Build history of the part. All positions in model axes, mm. Face numbers are marked on the shaded views. A direction names the side the tool comes from. Coordinates: 2 decimals unless noted, no trailing zeros. Order: outer loops, then holes, each group sorted by start corner. A loop starts at its lowest first (then second) coordinate and runs counter-clockwise, first axis right, second up. Notation, with made-up numbers: (-14, -15.75) - (28, -15.75) arc R26 cw to (28, 4.25) - close; hole circle Ø3 at (-17.75, 77.25). An arc over 180 degrees is marked (long way). Return JSON: item names as keys, results as strings.
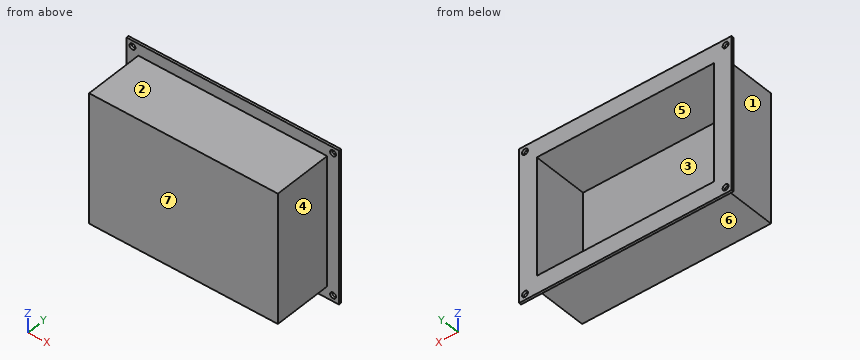
from build123d import *

# Parameters (mm, degrees)
SKETCH1_W                   = 203.2
SKETCH1_H                   = 139.7
BOSS_EXTRUDE2_DEPTH         = 63.5
SKETCH3_W                   = 228.6
SKETCH3_H                   = 165.1
BOSS_EXTRUDE3_DEPTH         = 2.54
F_1_4_0_25_DIAMETER_HOLE1_D = 6.35
SKETCH10_W                  = 190.5
SKETCH10_H                  = 127
CUT_EXTRUDE1_DEPTH          = 59.69


with BuildPart() as part:
    # Sketch1 → Boss-Extrude2 (new body)
    with BuildSketch(Plane(origin=(0, 0, 0), x_dir=(1, 0, 0), z_dir=(0, 1, 0))):
        Rectangle(SKETCH1_W, SKETCH1_H)
    extrude(amount=BOSS_EXTRUDE2_DEPTH)

    # Sketch3 → Boss-Extrude3 (add)
    with BuildSketch(Plane(origin=(0, 63.5, 0), x_dir=(1, 0, 0), z_dir=(0, 1, 0))):
        Rectangle(SKETCH3_W, SKETCH3_H)
    extrude(amount=BOSS_EXTRUDE3_DEPTH)

    # 1/4 (0.25) Diameter Hole1 (through all)
    with Locations(Plane(origin=(107.95, 63.5, -76.2), x_dir=(0, 0, -1), z_dir=(0, -1, 0))):
        with Locations((0, 0), (-152.4, 0), (0, -215.9), (-152.4, -215.9)):
            Hole(F_1_4_0_25_DIAMETER_HOLE1_D / 2)

    # Sketch10 → Cut-Extrude1 (cut)
    with BuildSketch(Plane(origin=(0, 66.04, 0), x_dir=(1, 0, 0), z_dir=(0, 1, 0))):
        Rectangle(SKETCH10_W, SKETCH10_H)
    extrude(amount=-CUT_EXTRUDE1_DEPTH, mode=Mode.SUBTRACT)


solid = part.part
1. Cut at D-D on z = -9. Give the cut face in (x, y), plus the area to 3 significant figures.
Check values:
{"outline": "(-114.3, 63.5) - (-101.6, 63.5) - (-101.6, 0) - (101.6, 0) - (101.6, 63.5) - (114.3, 63.5) - (114.3, 66.04) - (95.25, 66.04) - (95.25, 6.35) - (-95.25, 6.35) - (-95.25, 66.04) - (-114.3, 66.04) - close", "area": "2,110 mm²"}
2. Cut at A-A on y = 25.5. Give the cut face in (x, z), plus the area to 3 significant figures.
Check values:
{"outline": "(-101.6, -69.85) - (101.6, -69.85) - (101.6, 69.85) - (-101.6, 69.85) - close; hole (-95.25, -63.5) - (95.25, -63.5) - (95.25, 63.5) - (-95.25, 63.5) - close", "area": "4,190 mm²"}
3. Cut at C-C on z = -76.2. Give the cut face in (x, y) (3 decimals), plus the area to 3 significant figures.
Check values:
{"outline": "(-114.3, 63.5) - (-111.125, 63.5) - (-111.125, 66.04) - (-114.3, 66.04) - close; (-104.775, 63.5) - (104.775, 63.5) - (104.775, 66.04) - (-104.775, 66.04) - close; (111.125, 63.5) - (114.3, 63.5) - (114.3, 66.04) - (111.125, 66.04) - close", "area": "548 mm²"}
4. Probe L1, parallel to X at y = 64.15, z = -76.2 (3 decimals); L2, parallel to X at y = 56.5, z = -9; L3, parallel to Z at x = -107, y = 64. List the from-to ranges inside material, lowest first.
Check values:
{"L1": "-114.3 to -111.125, -104.775 to 104.775, 111.125 to 114.3", "L2": "-101.6 to -95.25, 95.25 to 101.6", "L3": "-82.55 to -79.23, -73.17 to 73.17, 79.23 to 82.55"}
5. Mould opens along X. For the marked faces 1, 2, 3 and 4 say: pulls with the +X half, pulls with the -X half, needs draft (parallel to the pull), parting line crosses it, or undercut.
Check values:
{"face 1": "pulls with the -X half", "face 2": "needs draft", "face 3": "undercut", "face 4": "pulls with the +X half"}
6. Tool access for the marked faces 5, 6 and 7: list every direction of +Z, -Z, +X, -X, +Y, -Y with a clear straight run to the whole face (end or side of a thin tool).
Check values:
{"face 5": "+Y", "face 6": "-Z, +X, -X, -Y", "face 7": "+Z, -Z, +X, -X, -Y"}
7. Drop flat-ended pins along their axis: pin 1 (5 mm diameter, centred on x = 107.95, z = -76.2, fed in from +Y); pin 2 (2 mm diameter, centred on x = -7, y = 19, fed in from +Z); pin 3 (5 mm diameter, centred on y = 14, z = 32, fed in from -X); pin 4 (3 mm diameter, centred on x = 13.5, y = 11, fed in from -Z). Give the stop position or say it passes through.
Check values:
{"pin 1": "through", "pin 2": "z = 69.85", "pin 3": "x = -101.6", "pin 4": "z = -69.85"}
8. Cut at B-B on x = 81. Give the cut face in (y, z).
Check values:
{"outline": "(0, -69.85) - (63.5, -69.85) - (63.5, -82.55) - (66.04, -82.55) - (66.04, -63.5) - (6.35, -63.5) - (6.35, 63.5) - (66.04, 63.5) - (66.04, 82.55) - (63.5, 82.55) - (63.5, 69.85) - (0, 69.85) - close"}
